Check sheet for the modelled part. Datum: model origin and axes. Units: mm. A direction names the side the tool comes from. Round coordinates to 2 decimals unless told otherwise and drop trailing zeros. Write each loop counter-clockwise with the first axis right and the second up, starting at its lowest first coordinate (ties: lowest second). Pieces come first, ordered by that corner, then holes. Notation, with made-up numbers: (43, 89.5) -> (77, 89.5) arc R19 cw to (77, 116.5) -> close; hole circle Ø5 at (34.25, 6). An arc over 180 degrees is marked (long way). Use one line per item in the form item = value. Start each with the question number.
```python
from build123d import *

# Parameters (mm, degrees)
BOSS_EXTRUDE1_DEPTH     = 10
SKETCH3_R               = 4
CUT_EXTRUDE1_DEPTH      = 20
SKETCH4_R               = 4
CUT_EXTRUDE2_DEPTH      = 10
SKETCH5_W               = 17
SKETCH5_H               = 18.5
CUT_EXTRUDE3_DEPTH      = 10
CUT_EXTRUDE3_DEPTH_BACK = 8.5


with BuildPart() as part:
    # Sketch1 → Boss-Extrude1 (new body, symmetric)
    with BuildSketch(Plane.XY):
        Polygon((-10, 0), (10, 0), (-10, 20), align=None)
    extrude(amount=BOSS_EXTRUDE1_DEPTH, both=True)

    # Sketch3 → Cut-Extrude1 (cut)
    with BuildSketch(Plane(origin=(0, 0, 0), x_dir=(1, 0, 0), z_dir=(0, 1, 0))):
        Circle(SKETCH3_R)
    extrude(amount=CUT_EXTRUDE1_DEPTH, mode=Mode.SUBTRACT)

    # Sketch4 → Cut-Extrude2 (cut, symmetric)
    with BuildSketch(Plane(origin=(0, 0, 0), x_dir=(0, 0, -1), z_dir=(1, 0, 0))):
        with Locations((0, 10)):
            Circle(SKETCH4_R)
    extrude(amount=CUT_EXTRUDE2_DEPTH, both=True, mode=Mode.SUBTRACT)

    # Sketch5 → Cut-Extrude3 (cut, two sides)
    with BuildSketch(Plane(origin=(0, 0, 0), x_dir=(0, 0, -1), z_dir=(1, 0, 0))) as cut_extrude3_sk:
        with Locations((0, 10.75)):
            Rectangle(SKETCH5_W, SKETCH5_H)
    extrude(amount=CUT_EXTRUDE3_DEPTH, mode=Mode.SUBTRACT)
    extrude(cut_extrude3_sk.sketch, amount=-CUT_EXTRUDE3_DEPTH_BACK, mode=Mode.SUBTRACT)


solid = part.part
```
1. Sectioned sample at B-B (z = 0). Enter the section's corners in (x, y).
2. Sectioned sample at C-C (x = 0). Enter the section's corners in (y, z).
3. Mould release check, pull along X, two halves, no side actions. Record for faces 3 (the face through (-4, 6, -8.5)), 4 (the face through (-8.5, 8, -4)), 5 (the face through (-0.867, 0.74, 3.905)): +X half, -X half, draft (parallel to the pull), parting line (faces both ways), or undercut.
4. Sectioned sample at A-A (y = 10). Enter the section's corners in (x, z), and give its area (3 significant figures).
5. Sectioned sample at D-D (y = 4.5). Enter the section's corners in (x, z).
6. Tool access check on faces 1 (the face through (-2, 1.5, -4)), 2 (the face through (-9.24, 13.966, 0.521)). Record the directions out of +Z, -Z, +X, -X, +Y, -Y that give a thin tool (end or side, any length) a straight path to the whole face; none if there is none.
7. Depth check by flat-ended pin: pin 1 (1 mm diameter, centred on y = 4, z = 7.5, fed in from +X); pin 2 (8 mm diameter, centred on y = 15, z = 7.5, fed in from +X); pin 3 (5 mm diameter, centred on x = -2, z = 4.5, fed in from +Y). Enter the tip coordinate at first touch or a pass-through.
8. Scan lines: probe 1 along Z at (x, y) = (0, 1.1); probe 2 along Z at (x, y) = (-1.75, 5); probe 3 along Y at (x, z) = (7, 6.25). Record each from-to range of solid material in increasing order.
Returned:
q1.outline = (-10, 0) -> (-4, 0) -> (-4, 1.5) -> (-8.5, 1.5) -> (-8.5, 6) -> (-10, 6) -> close; (-10, 14) -> (-8.5, 14) -> (-8.5, 18.5) -> (-10, 20) -> close; (4, 0) -> (10, 0) -> (8.5, 1.5) -> (4, 1.5) -> close
q2.outline = (0, -10) -> (10, -10) -> (10, -8.5) -> (1.5, -8.5) -> (1.5, -4) -> (0, -4) -> close; (0, 4) -> (1.5, 4) -> (1.5, 8.5) -> (10, 8.5) -> (10, 10) -> (0, 10) -> close
q3.face_3 = draft
q3.face_4 = +X half
q3.face_5 = undercut
q4.outline = (-10, -10) -> (0, -10) -> (0, -8.5) -> (-8.5, -8.5) -> (-8.5, -4) -> (-10, -4) -> close; (-10, 4) -> (-8.5, 4) -> (-8.5, 8.5) -> (0, 8.5) -> (0, 10) -> (-10, 10) -> close
q4.area = 43.5 mm^2
q5.outline = (-10, -10) -> (5.5, -10) -> (5.5, -8.5) -> (-8.5, -8.5) -> (-8.5, 8.5) -> (5.5, 8.5) -> (5.5, 10) -> (-10, 10) -> close
q6.face_1 = +X, +Y
q6.face_2 = +X, -X
q7.pin_1 = -8.5
q7.pin_2 = -1.13
q7.pin_3 = 1.5
q8.probe_1 = -10 to -4, 4 to 10
q8.probe_2 = -10 to -8.5, 8.5 to 10
q8.probe_3 = 0 to 1.5
